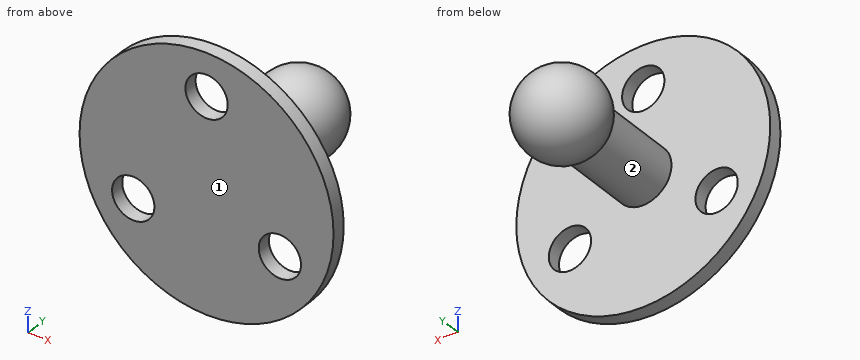
```python
from build123d import *

# Parameters (mm, degrees)
F0_R     = 14.2875
F0_R_2   = 2.38125
F1_DEPTH = 1.5875


with BuildPart() as f1:
    # F0 (on Front) → F1 (new body)
    with BuildSketch(Plane.XZ):
        Circle(F0_R)
        with Locations((-8.248891971, -4.7625)):
            Circle(F0_R_2, mode=Mode.SUBTRACT)
        with Locations((8.248891971, -4.7625)):
            Circle(F0_R_2, mode=Mode.SUBTRACT)
        with Locations((0, 9.525)):
            Circle(F0_R_2, mode=Mode.SUBTRACT)
    extrude(amount=F1_DEPTH)

    # F2 (on Top) → F3 (revolve)
    with BuildSketch(Plane.XY):
        with BuildLine():
            Line((0, 0), (3.175, 0))
            Line((3.175, 0), (3.175, 9.1502420857))
            ThreePointArc((3.175, 9.1502420857), (1.6993652025, 8.2510041404), (0, 7.9375))
            Line((0, 7.9375), (0, 0))
        make_face()
        with BuildLine():
            ThreePointArc((0, 7.9375), (1.6993652025, 8.2510041404), (3.175, 9.1502420857))
            ThreePointArc((3.175, 9.1502420857), (4.4489958596, 14.3993652025), (0, 17.4625))
            Line((0, 17.4625), (0, 12.7))
            Line((0, 12.7), (0, 7.9375))
        make_face()
    revolve(axis=Axis((0, 6.35, 0), (0, -1, 0)))


solid = f1.part
```
Geometry check sheet. Reference: the model listing, model coordinates, mm. Face numbers are marked on the shaded views. Coordinates: 2 decimals unless noted, no trailing zeros. Order: outer loops, then holes, each group sorted by start corner. A loop starts at its lowest first (then second) coordinate and runs counter-clockwise, first axis right, second up. Notation, with made-up numbers: (-20, -21) - (-8, -21) arc R12 ccw to (-8, -4) - close; hole circle Ø5 at (61.5, 37.25). An arc over 180 degrees is marked (long way). Answer as a JSON object with one key per item and string values. Group by question number.
Item 1: Sectioned sample at B-B, the plane z = 0. Record the cut outline in (x, y) (1 decimal).
Item 2: Scan lines: probe 1 along Z at (x, y) = (0, -0.5); probe 2 along Y at (x, z) = (-5.25, 13); probe 3 along Y at (x, z) = (2.5, 3.5). Record each from-to range of solid material in increasing order.
Item 3: Sectioned sample at C-C, the plane z = -5.5. Record the cut outline in (x, y).
Item 4: Draft check along Y on the marked faces 1 and 2. Enter one of: +Y half, -Y half, draft (parallel to the pull), parting line (faces both ways), or undercut.
Item 5: Sectioned sample at D-D, the plane y = 3.5. Record the cut outline in (x, z) (3 decimals).
Item 6: Depth check by flat-ended pin: pin 1 Ø10 at (x, y) = (-0.5, 5.5) entering from -Z; pin 2 Ø8 at (x, y) = (9, 2) entering from +Z; pin 3 Ø5.5 at (x, z) = (0, 9.525) entering from +Y; pin 4 Ø10 at (x, y) = (9.5, 5.5) entering from +Z. Enter the tip coordinate at first touch or a pass-through.
Item 7: Sectioned sample at A-A, the plane x = 0. Record the cut outline in (y, z) (1 decimal), and give its area (3 significant figures).
Resolved:
{
 "1": {"outline": "(-14.3, -1.6) - (14.3, -1.6) - (14.3, 0) - (3.2, 0) - (3.2, 9.2) arc R4.8 ccw (long way) to (-3.2, 9.2) - (-3.2, 0) - (-14.3, 0) - close"},
 "2": {"probe 1": "-14.29 to 7.14, 11.91 to 14.29", "probe 2": "-1.59 to 0", "probe 3": "-1.59 to 0, 10.66 to 14.74"},
 "3": {"outline": "(-13.19, -1.59) - (-10.51, -1.59) - (-10.51, 0) - (-13.19, 0) - close; (-5.98, -1.59) - (5.98, -1.59) - (5.98, 0) - (-5.98, 0) - close; (10.51, -1.59) - (13.19, -1.59) - (13.19, 0) - (10.51, 0) - close"},
 "4": {"face 1": "-Y half", "face 2": "undercut"},
 "5": {"outline": "circle Ø6.35 at (0, 0)"},
 "6": {"pin 1": "z = -4.21", "pin 2": "z = 13.17", "pin 3": "y = 0", "pin 4": "through"},
 "7": {"outline": "(-1.6, -14.3) - (0, -14.3) - (0, -3.2) - (9.2, -3.2) arc R4.8 ccw (long way) to (9.2, 3.2) - (0, 3.2) - (0, 7.1) - (-1.6, 7.1) - close; (-1.6, 11.9) - (0, 11.9) - (0, 14.3) - (-1.6, 14.3) - close", "area": "162 mm^2"}
}
